Part model, mm, in its own coordinate system. A direction names the side the tool comes from. Round coordinates to 2 decimals unless told otherwise and drop trailing zeros. Write each loop counter-clockwise with the first axis right and the second up, starting at its lowest first coordinate (ties: lowest second). Pieces come first, ordered by that corner, then holes.
1) Saw through at D-D on y = 6.5. Write the cut outline in (x, z).
2) Saw through at C-C on x = 8. Write the cut outline in (y, z), and give its area (3 significant figures).
3) Pull direction X, two halves, no side cores. Call faces 1 (the cylindrical face through (-8.195, -5.379, 4.93)), 2 (the cylindrical face through (31.816, -0.086, 4.93)), 3 (the flat face through (-25.38, -5.98, 4.93)): +X half, -X half, draft (parallel to the pull), parting line (faces both ways), or undercut.
4) Which spindle directions (+Z, -Z, +X, -X, +Y, -Y) get a long thin tool onto all of the face, cutting with end or side? Do faces 4 (the cylindrical face through (5.6, 6.93, 4.93)), 5 (the flat face through (5, -3, 5)), 6 (the cylindrical face through (8.415, -5.298, 4.93)). Say none if no direction does.
5) Drill centre lines: L1, parallel to Y at x = 8, z = 4; L2, parallel to X at y = -2.5, z = 3.5; L3, parallel to X at y = -0.75, z = 8.5. Where is each one in solid material? Low to high.
6) Flat gauge pins, fed straight in: pin 1 (4.5 mm diameter, centred on y = -2.5, z = 7, fed in from +X); pin 2 (4.5 mm diameter, centred on y = 4, z = 7, fed in from +X); pin 3 (4.5 mm diameter, centred on y = -3.5, z = 6, fed in from -X). Where does each tip first touch, or does it go through?
7) Saw through at B-B on z = 9. Count the separate pieces of the cut face and the enclosed holes in it, and give its area (3 significant figures).
8) Saw through at A-A on y = 0. Write the cut outline in (x, z), and give its area (3 significant figures).
```python
from build123d import *

# Parameters (mm, degrees)
SKETCH_R  = 0.9
PAD_DEPTH = 10


with BuildPart() as part:
    # Sketch (on XY_Plane of Origin) → Pad (new body)
    with BuildSketch(Plane.XY):
        with BuildLine():
            ThreePointArc((5, -5.5), (5.585786, -6.914214), (7, -7.5))
            Line((7, -7.5), (20.5, -7.5))
            ThreePointArc((20.5, -7.5), (21.413382, -7.415865), (22.296025, -7.166293))
            Line((22.296025, -7.166293), (28.548858, -4.759619))
            ThreePointArc((28.548858, -4.759619), (31.816912, 0), (28.548858, 4.759619))
            Line((28.548858, 4.759619), (22.296025, 7.166293))
            ThreePointArc((22.296025, 7.166293), (21.413382, 7.415865), (20.5, 7.5))
            Line((20.5, 7.5), (7, 7.5))
            ThreePointArc((7, 7.5), (5.585786, 6.914214), (5, 5.5))
            Line((5, 5.5), (5, 1.5))
            Line((-5, 1.5), (5, 1.5))
            Line((-5, 5.5), (-5, 1.5))
            ThreePointArc((-5, 5.5), (-5.585786, 6.914214), (-7, 7.5))
            Line((-20.5, 7.5), (-7, 7.5))
            ThreePointArc((-20.5, 7.5), (-21.413382, 7.415865), (-22.296025, 7.166293))
            Line((-28.548858, 4.759619), (-22.296025, 7.166293))
            ThreePointArc((-28.548858, 4.759619), (-31.816912, 0), (-28.548858, -4.759619))
            Line((-22.296025, -7.166293), (-28.548858, -4.759619))
            ThreePointArc((-22.296025, -7.166293), (-21.413382, -7.415865), (-20.5, -7.5))
            Line((-7, -7.5), (-20.5, -7.5))
            ThreePointArc((-7, -7.5), (-5.585786, -6.914214), (-5, -5.5))
            Line((-5, -1.5), (-5, -5.5))
            Line((-5, -1.5), (5, -1.5))
            Line((5, -1.5), (5, -5.5))
        make_face()
        with Locations((8, 4.5)):
            Circle(SKETCH_R, mode=Mode.SUBTRACT)
        with Locations((8, -4.5)):
            Circle(SKETCH_R, mode=Mode.SUBTRACT)
        with Locations((28.566912, 0)):
            Circle(SKETCH_R, mode=Mode.SUBTRACT)
        with Locations((-8, 4.5)):
            Circle(SKETCH_R, mode=Mode.SUBTRACT)
        with Locations((-8, -4.5)):
            Circle(SKETCH_R, mode=Mode.SUBTRACT)
        with Locations((-28.566912, 0)):
            Circle(SKETCH_R, mode=Mode.SUBTRACT)
    extrude(amount=PAD_DEPTH)


solid = part.part
```
Completed:
1. outline: (-24.03, 0) - (-5.27, 0) - (-5.27, 10) - (-24.03, 10) - close; (5.27, 0) - (24.03, 0) - (24.03, 10) - (5.27, 10) - close
2. outline: (-7.5, 0) - (-5.4, 0) - (-5.4, 10) - (-7.5, 10) - close; (-3.6, 0) - (3.6, 0) - (3.6, 10) - (-3.6, 10) - close; (5.4, 0) - (7.5, 0) - (7.5, 10) - (5.4, 10) - close
2. area: 114 mm2
3. face 1: undercut
3. face 2: +X half
3. face 3: -X half
4. face 4: +Z, -Z, +Y
4. face 5: +Z, -Z, -Y
4. face 6: +Z, -Z
5. L1: y = -7.5 to -5.4, -3.6 to 3.6, 5.4 to 7.5
5. L2: x = -31.16 to -5, 5 to 31.16
5. L3: x = -31.76 to -29.06, -28.07 to 28.07, 29.06 to 31.76
6. pin 1: stops at x = 31.81
6. pin 2: stops at x = 31.51
6. pin 3: stops at x = -31.66
7. separate pieces: 1
7. enclosed holes: 6
7. area: 724 mm2
8. outline: (-31.82, 0) - (-29.47, 0) - (-29.47, 10) - (-31.82, 10) - close; (-27.67, 0) - (27.67, 0) - (27.67, 10) - (-27.67, 10) - close; (29.47, 0) - (31.82, 0) - (31.82, 10) - (29.47, 10) - close
8. area: 600 mm2
